Check sheet for the modelled part. Datum: model origin and axes. Units: mm. Give positions to 0.01 mm unless a question says otherwise; leave off trailing zeros. Order: outer loops, then holes, each group sorted by start corner. A loop starts at its lowest first (then second) coordinate and runs counter-clockwise, first axis right, second up.
from build123d import *

# Parameters (mm, degrees)
MODEL_R                 = 1.105480949
SALIENTE_EXTRUIR1_DEPTH = 0.1


with BuildPart() as part:
    # Model → Saliente-Extruir1 (new body)
    with BuildSketch(Plane.XY):
        with BuildLine():
            Line((51.143384, -35.053134749), (51.143384, -20.385289094))
            ThreePointArc((51.143384, -20.385289094), (51.426053418, -19.68453986), (52.1199065, -19.385341948))
            Line((52.1199065, -19.385341948), (59.562610667, -19.385341948))
            Line((59.562610667, -19.385341948), (59.562610667, -17.385341948))
            Line((59.562610667, -17.385341948), (59.562610667, -16.385341948))
            Line((59.562610667, -16.385341948), (59.695317333, -16.385341948))
            ThreePointArc((59.695317333, -16.385341948), (65.261252438, -14.057943719), (67.588650667, -8.492008614))
            Line((67.588650667, -8.492008614), (67.463691144, 0.313086794))
            ThreePointArc((67.463691144, 0.313086794), (60.715005996, 0.09791285), (55.052059002, 3.775151269))
            Line((55.052059002, 3.775151269), (54.782677463, 27.772447041))
            ThreePointArc((54.782677463, 27.772447041), (60.525183262, 32.220247397), (67.588650667, 33.913389175))
            Line((67.588650667, 33.913389175), (67.588650667, 39.418409961))
            ThreePointArc((67.588650667, 39.418409961), (35.521984, 29.806750722), (3.455317333, 39.418409961))
            Line((3.455317333, 39.418409961), (3.545697938, 34.065337225))
            ThreePointArc((3.545697938, 34.065337225), (10.429922022, 32.177547893), (15.929001679, 27.626019279))
            Line((15.929001679, 27.626019279), (15.840502335, 3.627374762))
            ThreePointArc((15.840502335, 3.627374762), (10.205432608, -0.092442467), (3.455317333, 0.071858577))
            Line((3.455317333, 0.071858577), (3.455317333, -8.386134749))
            ThreePointArc((3.455317333, -8.386134749), (5.745129751, -14.020897609), (11.348650667, -16.386134749))
            Line((11.348650667, -16.386134749), (11.481357333, -16.386134749))
            Line((11.481357333, -16.386134749), (11.481357333, -19.386134749))
            Line((11.481357333, -19.386134749), (18.913917333, -19.386134749))
            ThreePointArc((18.913917333, -19.386134749), (19.614357448, -19.681789392), (19.900584, -20.386134749))
            Line((19.900584, -20.386134749), (19.900584, -35.053134749))
            Line((19.900584, -35.053134749), (31.411037333, -35.053134749))
            Line((31.411037333, -35.053134749), (31.411037333, -16.386134749))
            Line((31.411037333, -16.386134749), (39.632930667, -16.386134749))
            Line((39.632930667, -16.386134749), (39.632930667, -35.053134749))
            Line((39.632930667, -35.053134749), (51.143384, -35.053134749))
        make_face()
        Polygon((35.504038921, 26.200203798), (50.790705587, 26.200203798), (50.790705587, -5.799796202), (19.217372254, -5.799796202), (19.217372254, 26.200203798), align=None, mode=Mode.SUBTRACT)
        with Locations((18.402228125, 27.990495682)):
            Circle(MODEL_R, mode=Mode.SUBTRACT)
        with Locations((52.306774108, 28.11827167)):
            Circle(MODEL_R, mode=Mode.SUBTRACT)
    extrude(amount=SALIENTE_EXTRUIR1_DEPTH)


solid = part.part
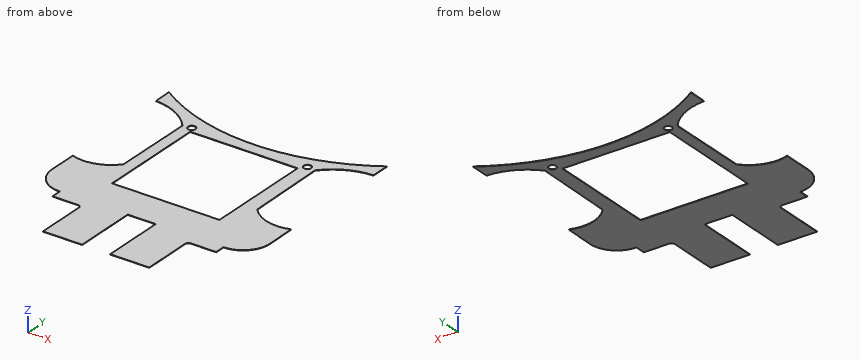
1) Section check B-B, the plane x = 26. Record the cut outline in (y, z), then the cut area to 3 significant figures.
Recorded:
outline: (-35.05, 0) - (-5.8, 0) - (-5.8, 0.1) - (-35.05, 0.1) - close; (26.2, 0) - (30.59, 0) - (30.59, 0.1) - (26.2, 0.1) - close
area: 3.36 mm2
2) Section check A-A, the plane y = -18. Record the cut outline in (x, z), then the cut area to 3 significant figures.
Recorded:
outline: (11.48, 0) - (31.41, 0) - (31.41, 0.1) - (11.48, 0.1) - close; (39.63, 0) - (59.56, 0) - (59.56, 0.1) - (39.63, 0.1) - close
area: 3.99 mm2
3) Depth check by flat-ended pin: pin 1 Ø3 at (x, y) = (52.31, 28.12) entering from +Z. Enter the tip coordinate at first touch or a pass-through.
Recorded:
pin 1: stops at z = 0.1
4) Material ranges on L1, parallel to X at y = 25, z = 0.05; L2, parallel to Y at x = 6, z = 0.05, recorded low to high.
Recorded:
L1: x = 15.92 to 19.22, 50.79 to 54.81
L2: y = -14.27 to -0.48, 33.75 to 37.83
5) Section check C-C, the plane z = 0.05. State how many separate pieces and enclosed holes the cut face has, then the cut area to 3 significant figures.
Recorded:
separate pieces: 1
enclosed holes: 3
area: 1,810 mm2
